```python
from build123d import *

# Parameters (mm, degrees)
SKETCH_1_W      = 75
SKETCH_1_H      = 695
EXTRUDE_1_DEPTH = 4
SKETCH_2_W      = 4
SKETCH_2_H      = 695
EXTRUDE_2_DEPTH = 36


with BuildPart() as part:
    # 스케치1 → 보스-돌출1 (new body)
    with BuildSketch(Plane.XY):
        with Locations((37.5, 347.5)):
            Rectangle(SKETCH_1_W, SKETCH_1_H)
    extrude(amount=EXTRUDE_1_DEPTH)

    # 스케치2 → 보스-돌출2 (add)
    with BuildSketch(Plane(origin=(0, 0, 0), x_dir=(-1, 0, 0), z_dir=(0, 0, -1))):
        with Locations((-73, 347.5)):
            Rectangle(SKETCH_2_W, SKETCH_2_H)
        with Locations((-2, 347.5)):
            Rectangle(SKETCH_2_W, SKETCH_2_H)
    extrude(amount=EXTRUDE_2_DEPTH)


solid = part.part
```
The model under review builds one solid part; all positions refer to its coordinate system, in mm. A direction names the side the tool comes from. Round coordinates to 2 decimals unless told otherwise and drop trailing zeros. Order: outer loops, then holes, each group sorted by start corner. A loop starts at its lowest first (then second) coordinate and runs counter-clockwise, first axis right, second up.
Item 1: Draft analysis for pull direction X (two halves, no side actions). For faces 3 (the flat face through (0, 343, -16)), 4 (the flat face through (43.2, 695, 0.4)), 5 (the flat face through (71, 343, -18)), state which applies: released by +X, released by -X, zero draft, split by the parting line, or undercut.
Working result:
face 3: released by -X
face 4: zero draft
face 5: undercut
Item 2: Add section C-C, the plane x = 52. State the section outline as (y, z) points, and give its area (3 significant figures).
Working result:
outline: (0, 0) - (695, 0) - (695, 4) - (0, 4) - close
area: 2,780 mm2
Item 3: For pin 1 (20 mm diameter, centred on x = 34, y = 388.5, fed in from -Z), flat-tipped, find the tip position at first contact; note if it passes through.
Working result:
pin 1: stops at z = 0
Item 4: Machinability: for faces 1 (the flat face through (37, 352, 0)), 2 (the flat face through (43.2, 0, 0.4)), which of the approach directions +Z, -Z, +X, -X, +Y, -Y give a long, thin tool a straight path to every point of the face, cutting with its end or side? Answer none if there is none.
Working result:
face 1: -Z, +Y, -Y
face 2: +Z, -Z, +X, -X, -Y
Item 5: Add section B-B, the plane y = 493.5. State the section outline as (x, z) points, and give its area (3 significant figures).
Working result:
outline: (0, -36) - (4, -36) - (4, 0) - (71, 0) - (71, -36) - (75, -36) - (75, 4) - (0, 4) - close
area: 588 mm2
Item 6: Add section A-A, the plane z = -11.5. State the section outline as (x, y) points.
Working result:
outline: (0, 0) - (4, 0) - (4, 695) - (0, 695) - close; (71, 0) - (75, 0) - (75, 695) - (71, 695) - close
Item 7: To check wall thickness, follow probe 1 along X at (y, z) = (416.5, -21.5); probe 2 along Z at (x, y) = (38, 157). State the ranges of each line that lie inside material, in increasing order.
Working result:
probe 1: x = 0 to 4, 71 to 75
probe 2: z = 0 to 4
